from build123d import *

# Parameters (mm, degrees)
F0_R      = 15
F1_DEPTH  = 1500
F2_R      = 13.75
F3_DEPTH  = 3000
F7_DEPTH  = 10
F9_DEPTH  = 10
F12_R     = 22.5
F13_DEPTH = 200
F14_SIZE  = 5


with BuildPart() as f1:
    # F0 (on Front) → F1 (new body)
    with BuildSketch(Plane.XZ):
        Circle(F0_R)
    extrude(amount=-F1_DEPTH)

    # F2 (on face) → F3 (cut)
    with BuildSketch(Plane.XZ):
        Circle(F2_R)
    extrude(amount=-F3_DEPTH, mode=Mode.SUBTRACT)

    # F6 (on offset) → F7 (cut)
    with BuildSketch(Plane.YZ.offset(15)):
        Polygon((30, 5), (0, 5), (0, -1), (22, -1), (22, -11), (38, -11), (38, -5), (30, -5), align=None)
    extrude(amount=-F7_DEPTH, mode=Mode.SUBTRACT)

    # F8 (on offset) → F9 (cut)
    with BuildSketch(Plane.YZ.offset(-15)):
        Polygon((22, 1), (0, 1), (0, -5), (30, -5), (30, 5), (38, 5), (38, 11), (22, 11), align=None)
    extrude(amount=F9_DEPTH, mode=Mode.SUBTRACT)

    # F12 (on offset) → F13 (join)
    with BuildSketch(Plane.XZ.offset(-1200)):
        Circle(F12_R)
    extrude(amount=F13_DEPTH)

    # F14
    f14_edges = [f1.edges().sort_by_distance(p)[0] for p in [
        (22.5, 1100, 0),
        (-22.5, 1200, 0),
        (-22.5, 1000, 0),
    ]]
    chamfer(f14_edges, length=F14_SIZE)


solid = f1.part
Can you work these out from the model? Positions are in its coordinate system, mm. A direction names the side the tool comes from. Coordinates: 2 decimals unless noted, no trailing zeros. Loops run counter-clockwise (first coordinate to the right, second up) from the corner with the lowest first, then second, coordinate; pieces in that order, holes last. Notation, with made-up numbers: (54.25, 10) - (100.25, 10) arc R23 cw to (100.25, 28) - close; hole circle Ø11 at (35.5, 58.5). An arc over 180 degrees is marked (long way). Answer as a JSON object with one key per item and string values. Group by question number.
Item 1: If we section it at B-B (y = 799): List the corners of the cut face in (x, z) for me.
Item 2: If we section it at A-A (x = 0): List the corners of the cut face in (y, z) for me.
Item 3: On a 3-axis mill with a long thin cutter (end or side, diameter ignored), from which of +Z, -Z, +X, -X, +Y, -Y can I reach the whole of each face in a straight line? I mean faces 4 (the face through (4.4, 1500, -13.3)), 5 (the face through (-2.981, 493, -13.423)), 6 (the face through (13, 1200, 8)). Say none if no direction works.
Item 4: If we mould it in two halves opening along Z, with no side actions, what happens to faces 1 (the face through (10.382, 1101.33, -19.961)), 2 (the face through (-2.981, 1347.9, -13.423)), 3 (the face through (13, 1000, 8))? For each: released by +Z, released by -Z, zero draft, split by the parting line, or undercut.
Item 5: If I drill on L1, parallel to Z at x = 0, y = 1363.5; L2, parallel to X at y = 433.5, z = -5.5, over which ranges is the centre line in solid material (lowest first)? Write a range as from..to.
Item 6: For pin 1 (1.1 mm diameter, centred on x = -13.5, z = -0.5, fed in from -Y); pin 2 (10 mm diameter, centred on x = 0, y = 620.5, fed in from +Z); pin 3 (10 mm diameter, centred on y = 787.5, z = 9.5, fed in from +X), each with a flat end and sliding along its axis, tell me the tip position at first contact or that it passes through.
Returned:
{
 "1": {"outline": "circle Ø30 at (0, 0); hole circle Ø27.5 at (0, 0)"},
 "2": {"outline": "(0, -15) - (1000, -15) - (1000, -17.5) - (1005, -22.5) - (1195, -22.5) - (1200, -17.5) - (1200, -15) - (1500, -15) - (1500, -13.75) - (1200, -13.75) - (1200, 13.75) - (1500, 13.75) - (1500, 15) - (1200, 15) - (1200, 17.5) - (1195, 22.5) - (1005, 22.5) - (1000, 17.5) - (1000, 15) - (0, 15) - (0, 13.75) - (1000, 13.75) - (1000, -13.75) - (0, -13.75) - close"},
 "3": {"face 4": "+Z, -Z, +X, -X, +Y", "face 5": "-Y", "face 6": "+Y"},
 "4": {"face 1": "split by the parting line", "face 2": "undercut", "face 3": "zero draft"},
 "5": {"L1": "z = -15..-13.75, 13.75..15", "L2": "x = -13.96..-12.6, 12.6..13.96"},
 "6": {"pin 1": "stops at y = 30", "pin 2": "stops at z = 15", "pin 3": "stops at x = 14.31"}
}
